Check sheet for the modelled part. Datum: model origin and axes. Units: mm. Round coordinates to 2 decimals unless told otherwise and drop trailing zeros. Order: outer loops, then holes, each group sorted by start corner. A loop starts at its lowest first (then second) coordinate and runs counter-clockwise, first axis right, second up. Notation, with made-up numbers: (70, 6.25) -> (74, 6.25) arc R34 cw to (74, 40.25) -> close; hole circle Ø4 at (-30, -14). An arc over 180 degrees is marked (long way). Answer in a Markdown table with one row per item.
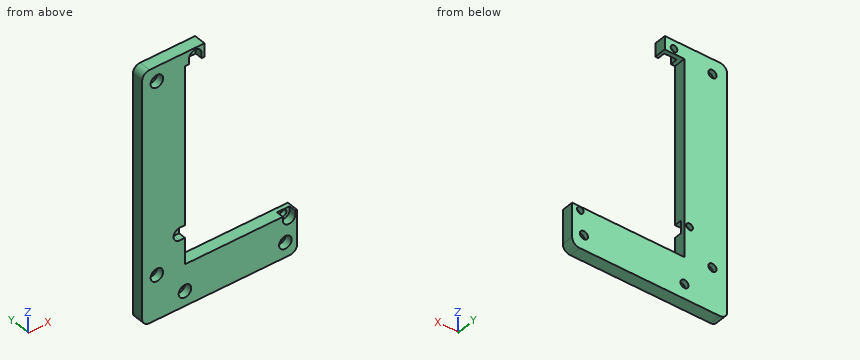
from build123d import *

# Parameters (mm, degrees)
SKETCH2_R                = 2.75
SKETCH2_R_2              = 2.25
BOSS_EXTRUDE1_DEPTH      = 4
BOSS_EXTRUDE1_DEPTH_BACK = 4
SKETCH3_R                = 4.25
CUT_EXTRUDE1_DEPTH       = 5


with BuildPart() as part:
    # Sketch2 → Boss-Extrude1 (new body, two sides)
    with BuildSketch(Plane(origin=(0, 0, 0), x_dir=(1, 0, 0), z_dir=(0, 1, 0))) as boss_extrude1_sk:
        with BuildLine():
            ThreePointArc((-52.5, -80), (-51.035533906, -83.535533906), (-47.5, -85))
            Line((-47.5, -85), (-23.5, -85))
            Line((-23.5, -85), (-10.25, -85))
            Line((-10.25, -85), (-10.25, -76))
            Line((-10.25, -76), (-23.5, -76))
            Line((-23.5, -76), (-23.5, -62.428663753))
            Line((-23.5, -62.428663753), (-23.5, 57))
            Line((-23.5, 57), (52.5, 57))
            Line((52.5, 57), (52.5, 80))
            ThreePointArc((52.5, 80), (51.035533906, 83.535533906), (47.5, 85))
            Line((47.5, 85), (-47.5, 85))
            ThreePointArc((-47.5, 85), (-51.035533906, 83.535533906), (-52.5, 80))
            Line((-52.5, 80), (-52.5, -80))
        make_face()
        with Locations((-42.5, -75)):
            Circle(SKETCH2_R, mode=Mode.SUBTRACT)
        with Locations((-16.5, -79.5)):
            Circle(SKETCH2_R_2, mode=Mode.SUBTRACT)
        with Locations((-27, 35)):
            Circle(SKETCH2_R_2, mode=Mode.SUBTRACT)
        with Locations((-42.5, 55)):
            Circle(SKETCH2_R, mode=Mode.SUBTRACT)
        with Locations((-23.5, 75)):
            Circle(SKETCH2_R, mode=Mode.SUBTRACT)
        with Locations((47, 59.5)):
            Circle(SKETCH2_R_2, mode=Mode.SUBTRACT)
        with Locations((44.5, 75)):
            Circle(SKETCH2_R, mode=Mode.SUBTRACT)
    extrude(amount=BOSS_EXTRUDE1_DEPTH)
    extrude(boss_extrude1_sk.sketch, amount=-BOSS_EXTRUDE1_DEPTH_BACK)

    # Sketch3 → Cut-Extrude1 (cut)
    with BuildSketch(Plane.XZ.offset(4)):
        with Locations((-23.5, -75)):
            Circle(SKETCH3_R)
        with Locations((-42.5, -55)):
            Circle(SKETCH3_R)
        with Locations((-42.5, 75)):
            Circle(SKETCH3_R)
        with Locations((44.5, -75)):
            Circle(SKETCH3_R)
        with BuildLine():
            Line((-27, -30.75), (-23.5, -30.75))
            Line((-23.5, -30.75), (-23.5, -39.25))
            Line((-23.5, -39.25), (-27, -39.25))
            ThreePointArc((-27, -39.25), (-31.25, -35), (-27, -30.75))
        make_face()
        with BuildLine():
            Line((51.25, -59.5), (51.25, -57))
            Line((51.25, -57), (42.75, -57))
            Line((42.75, -57), (42.75, -59.5))
            ThreePointArc((42.75, -59.5), (47, -63.75), (51.25, -59.5))
        make_face()
        with BuildLine():
            Line((-12.25, 79.5), (-12.25, 76))
            Line((-12.25, 76), (-20.75, 76))
            Line((-20.75, 76), (-20.75, 79.5))
            ThreePointArc((-20.75, 79.5), (-16.5, 83.75), (-12.25, 79.5))
        make_face()
    extrude(amount=-CUT_EXTRUDE1_DEPTH, mode=Mode.SUBTRACT)


solid = part.part
Item 1: Cross-section at A-A (x = -42.5). Record the boundary of the cut face in (y, z), and give its area (3 significant figures).
Result sheet:
| item | result |
|---|---|
| outline | (-4, -85) -> (4, -85) -> (4, -57.75) -> (1, -57.75) -> (1, -59.25) -> (-4, -59.25) -> close; (-4, -50.75) -> (1, -50.75) -> (1, -52.25) -> (4, -52.25) -> (4, 72.25) -> (1, 72.25) -> (1, 70.75) -> (-4, 70.75) -> close; (-4, 79.25) -> (1, 79.25) -> (1, 77.75) -> (4, 77.75) -> (4, 85) -> (-4, 85) -> close |
| area | 1,240 mm^2 |
Item 2: Cross-section at D-D (x = -16.5). Record the boundary of the cut face in (y, z).
Result sheet:
| item | result |
|---|---|
| outline | (-4, -85) -> (4, -85) -> (4, -57) -> (-4, -57) -> close; (-4, 83.75) -> (1, 83.75) -> (1, 81.75) -> (4, 81.75) -> (4, 85) -> (-4, 85) -> close; (1, 76) -> (4, 76) -> (4, 77.25) -> (1, 77.25) -> close |
Item 3: Cross-section at B-B (y = -2.75). Record the boundary of the cut face in (x, z), and give its area (3 significant figures).
Result sheet:
| item | result |
|---|---|
| outline | (-52.5, -80) arc R5 ccw to (-47.5, -85) -> (47.5, -85) arc R5 ccw to (52.5, -80) -> (52.5, -57) -> (51.25, -57) -> (51.25, -59.5) arc R4.25 cw to (42.75, -59.5) -> (42.75, -57) -> (-23.5, -57) -> (-23.5, -39.25) -> (-27, -39.25) arc R4.25 cw to (-27, -30.75) -> (-23.5, -30.75) -> (-23.5, 76) -> (-20.75, 76) -> (-20.75, 79.5) arc R4.25 cw to (-12.25, 79.5) -> (-12.25, 76) -> (-10.25, 76) -> (-10.25, 85) -> (-47.5, 85) arc R5 ccw to (-52.5, 80) -> close; hole circle Ø8.5 at (-42.5, -55); hole circle Ø8.5 at (-42.5, 75); hole circle Ø8.5 at (-23.5, -75); hole circle Ø8.5 at (44.5, -75) |
| area | 6,770 mm^2 |
Item 4: Cross-section at C-C (z = -75). Record the boundary of the cut face in (x, y), and give its area (3 significant figures).
Result sheet:
| item | result |
|---|---|
| outline | (-52.5, -4) -> (-27.75, -4) -> (-27.75, 1) -> (-26.25, 1) -> (-26.25, 4) -> (-52.5, 4) -> close; (-20.75, 1) -> (-19.25, 1) -> (-19.25, -4) -> (40.25, -4) -> (40.25, 1) -> (41.75, 1) -> (41.75, 4) -> (-20.75, 4) -> close; (47.25, 1) -> (48.75, 1) -> (48.75, -4) -> (52.5, -4) -> (52.5, 4) -> (47.25, 4) -> close |
| area | 722 mm^2 |
Item 5: Scan lines: line 1 (X direction, y = 3.2, z = -75); line 2 (X direction, y = -0.25, z = -75.5); line 3 (Z direction, x = -42.5, y = -2.35). Record each from-to range of solid material in increasing order. Write a range as [from, to].
Result sheet:
| item | result |
|---|---|
| line 1 | x = [-52.5, -26.25], [-20.75, 41.75], [47.25, 52.5] |
| line 2 | x = [-52.5, -27.72], [-19.28, 40.28], [48.72, 52.5] |
| line 3 | z = [-85, -59.25], [-50.75, 70.75], [79.25, 85] |
Item 6: Depth check by flat-ended pin: P1, Ø4, axis at y = 2, z = -37, coming from the +X side. Enter the tip coordinate at first touch or a pass-through.
Result sheet:
| item | result |
|---|---|
| P1 | stops at x = -23.5 |
